Can you work these out from the drawing? Everything is in mm from the part's minimum corner. Coordinates: 2 decimals unless noted, no trailing zeros. Write each loop counter-clockwise with the first axis right and the second up, starting at its lowest first coordinate (ties: lowest second). Pieces come first, ordered by that corner, then holes. Notation, with made-up numbers: M -29,76 L -10,76 A33 cw -10,111 Z; hole C -17,82.5 d11. An arc over 180 degrees is marked long. Write item = value, one per line.
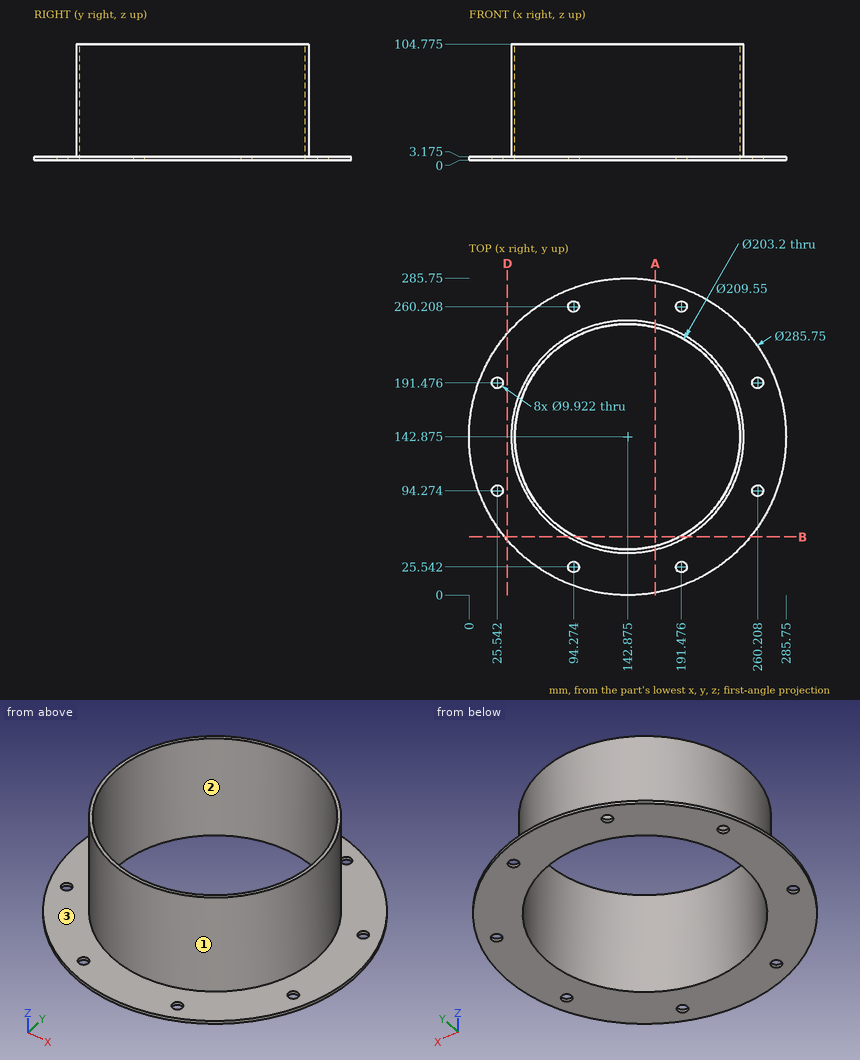
Item 1: If we mould it in two halves opening along X, with no side actions, what happens to the marked faces 1, 2 and 3? For each: pulls with the +X half, pulls with the -X half, needs draft (parallel to the pull), parting line crosses it, or undercut.
Numbers:
face_1 = parting line crosses it
face_2 = undercut
face_3 = needs draft
Item 2: Imagine slicing it at A-A (x = 168). Write out the boundary of the cut face in (y, z) (1 decimal).
Numbers:
outline = M 2.2,0 L 44.4,0 L 44.4,104.8 L 41.2,104.8 L 41.2,3.2 L 2.2,3.2 Z; M 241.3,0 L 283.5,0 L 283.5,3.2 L 244.6,3.2 L 244.6,104.8 L 241.3,104.8 Z
Item 3: Imagine slicing it at B-B (y = 52.5). Write out the boundary of the cut face in (x, z) (1 decimal), and give its area (3 significant figures).
Numbers:
outline = M 32.2,0 L 96.5,0 L 96.5,104.8 L 89.9,104.8 L 89.9,3.2 L 32.2,3.2 Z; M 189.3,0 L 253.5,0 L 253.5,3.2 L 195.9,3.2 L 195.9,104.8 L 189.3,104.8 Z
area = 1,750 mm²
Item 4: I'm going to push flat-ended pins straight in: P1, Ø8, axis at y = 47, z = 42, coming from the -X side; P2, Ø3, axis at x = 65, z = 39.5, coming from the +Y side; P3, Ø3, axis at x = 238.5, z = 72, coming from the +Y side. Where does each tip first touch, or does it pass through?
Numbers:
P1 = 92.51
P2 = 214.6
P3 = 188.9
Item 5: If I drill on line 1 along Y through (x, z) = (142.5, 44); line 2 along X through (y, z) = (227.5, 22); line 3 along Y through (x, z) = (69, 25) (1 decimal), over which ranges is the centre line in solid material (lowest first)?
Numbers:
line_1 = 38.1 to 41.28, 244.47 to 247.65
line_2 = 81.1 to 86.65, 199.1 to 204.65
line_3 = 68.6 to 73.1, 212.6 to 217.2
Item 6: Imagine slicing it at D-D (x = 34.5). Write out the boundary of the cut face in (y, z) (1 decimal), and give its area (3 significant figures).
Numbers:
outline = M 49.8,0 L 236,0 L 236,3.2 L 49.8,3.2 Z
area = 591 mm²
